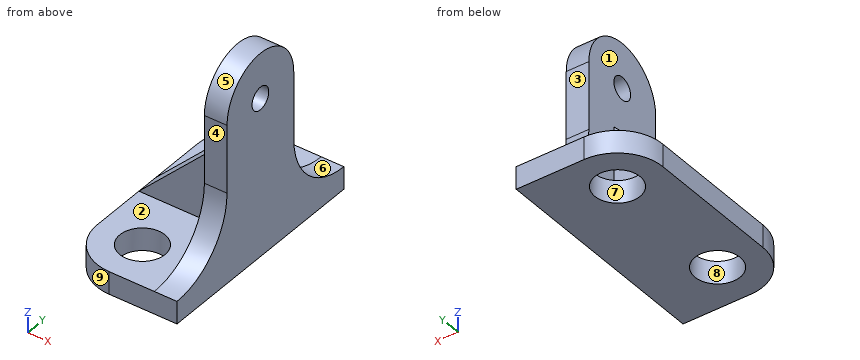
```python
from build123d import *

# Parameters (mm, degrees)
SKETCH002_R  = 5
PAD001_DEPTH = 5
SKETCH003_R  = 2.5
PAD002_DEPTH = 5
PAD003_DEPTH = 2.5


with BuildPart() as part:
    # Sketch002 → Pad001 (new body)
    with BuildSketch(Plane.XY):
        with BuildLine():
            Line((0, 25), (-15, 25))
            ThreePointArc((-15, 25), (-22.071068, 22.071068), (-25, 15))
            Line((-25, 15), (-25, -15))
            ThreePointArc((-25, -15), (-22.071068, -22.071068), (-15, -25))
            Line((-15, -25), (0, -25))
            Line((0, -25), (0, 25))
        make_face()
        with Locations((-15, 15)):
            Circle(SKETCH002_R, mode=Mode.SUBTRACT)
        with Locations((-15, -15)):
            Circle(SKETCH002_R, mode=Mode.SUBTRACT)
    extrude(amount=PAD001_DEPTH)

    # Sketch003 → Pad002 (join)
    with BuildSketch(Plane.YZ):
        with BuildLine():
            ThreePointArc((-25, 5), (-14.393398, 9.393398), (-10, 20))
            Line((-10, 20), (-10, 35))
            ThreePointArc((10, 35), (0, 45), (-10, 35))
            Line((10, 20), (10, 35))
            ThreePointArc((10, 20), (14.393398, 9.393398), (25, 5))
            Line((-25, 5), (25, 5))
        make_face()
        with Locations((0, 35)):
            Circle(SKETCH003_R, mode=Mode.SUBTRACT)
    extrude(amount=-PAD002_DEPTH)

    # Sketch004 → Pad003 (join, symmetric)
    with BuildSketch(Plane.XZ):
        Polygon((-25, 5), (-5, 5), (-5, 25), align=None)
    extrude(amount=PAD003_DEPTH, both=True)


solid = part.part
```
Input: part model. Units: mm. Frame: model coordinates. Face numbers are marked on the shaded views. A direction names the side the tool comes from. Round coordinates to 2 decimals unless told otherwise and drop trailing zeros. Loops run counter-clockwise (first coordinate to the right, second up) from the corner with the lowest first, then second, coordinate; pieces in that order, holes last.
1) Pin query (flat end, axial travel): pin 1 (12 mm diameter, centred on y = -5, z = 28, fed in from +X); pin 2 (4 mm diameter, centred on x = -4, y = 5.5, fed in from +Z); pin 3 (10 mm diameter, centred on x = -12, y = 8.5, fed in from +Z); pin 4 (1.5 mm diameter, centred on x = -3, y = -1, fed in from +Z). Return the tip coordinate at first contact, or that it passes through.
Ans:
pin 1: stops at x = 0
pin 2: stops at z = 44.37
pin 3: stops at z = 5
pin 4: stops at z = 45
2) Section query B-B on z = 8. Return the cut outline in (x, y), plus the area to 3 significant figures.
Ans:
outline: (-22, -2.5) - (-5, -2.5) - (-5, -16) - (0, -16) - (0, 16) - (-5, 16) - (-5, 2.5) - (-22, 2.5) - close
area: 245 mm2
3) Material intervals for line 1 (Y direction, x = -15, z = 3.3); line 2 (Z direction, x = -1.1, y = 0); line 3 (Z direction, x = -16, y = -21), sorted ascending.
Ans:
line 1: y = -25 to -20, -10 to 10, 20 to 25
line 2: z = 0 to 32.5, 37.5 to 45
line 3: z = 0 to 5
4) Set-up query: the marked faces 1, 2, 3, 4 and 5. Return all of +Z, -Z, +X, -X, +Y, -Y with unobstructed straight access to the full face (end or side cutting, diameter ignored); none if empty.
Ans:
face 1: +Z, -X
face 2: +Z, -X, -Y
face 3: +Z, +X, -X, +Y
face 4: +Z, +X, -X, -Y
face 5: +Z, +X, -X
5) Section query D-D on x = -16.5. Return the cut outline in (y, z), plus the area to 3 significant figures.
Ans:
outline: (-24.89, 0) - (-19.77, 0) - (-19.77, 5) - (-24.89, 5) - close; (-10.23, 0) - (10.23, 0) - (10.23, 5) - (2.5, 5) - (2.5, 13.5) - (-2.5, 13.5) - (-2.5, 5) - (-10.23, 5) - close; (19.77, 0) - (24.89, 0) - (24.89, 5) - (19.77, 5) - close
area: 196 mm2
6) Pull-direction query (X, two-part tool) for the marked faces 6, 7, 8 and 9; classes: released by +X, released by -X, zero draft, split by the parting line, or undercut.
Ans:
face 6: zero draft
face 7: undercut
face 8: undercut
face 9: released by -X
7) Section query A-A on y = 12. Return the cut outline in (x, z), plus the area to 3 significant figures.
Ans:
outline: (-25, 0) - (-19, 0) - (-19, 5) - (-25, 5) - close; (-11, 0) - (0, 0) - (0, 12.52) - (-5, 12.52) - (-5, 5) - (-11, 5) - close
area: 123 mm2
8) Section query C-C on x = -5.75. Return the cut outline in (y, z), plus the area to 3 significant figures.
Ans:
outline: (-25, 0) - (25, 0) - (25, 5) - (2.5, 5) - (2.5, 24.25) - (-2.5, 24.25) - (-2.5, 5) - (-25, 5) - close
area: 346 mm2
